Work out the finished part from the listing and answer in its coordinate system (mm). Coordinates: 2 decimals unless noted, no trailing zeros. Order: outer loops, then holes, each group sorted by start corner. A loop starts at its lowest first (then second) coordinate and runs counter-clockwise, first axis right, second up. Notation, with made-up numbers: M -34.75,-35.5 L 3.25,-35.5 A12 ccw 3.25,-16.5 Z; hole C 61,88 d7. An arc over 180 degrees is marked long. Use a Markdown table: item, result. Add a question column.
from build123d import *

# Parameters (mm, degrees)
SKETCH1_W           = 600
SKETCH1_H           = 300
BOSS_EXTRUDE1_DEPTH = 3
SKETCH2_R           = 82.5
SKETCH2_R_2         = 6.5
SKETCH2_W           = 30
SKETCH2_H           = 3
SKETCH2_W_2         = 3
SKETCH2_H_2         = 30
CUT_EXTRUDE2_DEPTH  = 5
SKETCH3_W           = 175.2
SKETCH3_H           = 3.2
CUT_EXTRUDE3_DEPTH  = 10


with BuildPart() as part:
    # Sketch1 → Boss-Extrude1 (new body)
    with BuildSketch(Plane(origin=(0, 0, 0), x_dir=(1, 0, 0), z_dir=(0, 1, 0))):
        with Locations((300, 150)):
            Rectangle(SKETCH1_W, SKETCH1_H)
    extrude(amount=BOSS_EXTRUDE1_DEPTH)

    # Sketch2 → Cut-Extrude2 (cut)
    with BuildSketch(Plane(origin=(0, 3, 0), x_dir=(1, 0, 0), z_dir=(0, 1, 0))):
        with Locations(Location((115, 150, 0), (0, 0, 270))):
            Circle(SKETCH2_R)
        with Locations(Location((263.5, 150, 0), (0, 0, 270))):
            Circle(SKETCH2_R_2)
        with Locations(Location((336.5, 150, 0), (0, 0, 90))):
            Circle(SKETCH2_R_2)
        with Locations(Location((485, 150, 0), (0, 0, 90))):
            Circle(SKETCH2_R)
        with Locations((90, 1.5)):
            Rectangle(SKETCH2_W, SKETCH2_H)
        with Locations((30, 1.5)):
            Rectangle(SKETCH2_W, SKETCH2_H)
        with Locations((150, 1.5)):
            Rectangle(SKETCH2_W, SKETCH2_H)
        with Locations((210, 1.5)):
            Rectangle(SKETCH2_W, SKETCH2_H)
        with Locations((270, 1.5)):
            Rectangle(SKETCH2_W, SKETCH2_H)
        with Locations((330, 1.5)):
            Rectangle(SKETCH2_W, SKETCH2_H)
        with Locations((390, 1.5)):
            Rectangle(SKETCH2_W, SKETCH2_H)
        with Locations((450, 1.5)):
            Rectangle(SKETCH2_W, SKETCH2_H)
        with Locations((510, 1.5)):
            Rectangle(SKETCH2_W, SKETCH2_H)
        with Locations((570, 1.5)):
            Rectangle(SKETCH2_W, SKETCH2_H)
        with Locations((570, 298.5)):
            Rectangle(SKETCH2_W, SKETCH2_H)
        with Locations((510, 298.5)):
            Rectangle(SKETCH2_W, SKETCH2_H)
        with Locations((450, 298.5)):
            Rectangle(SKETCH2_W, SKETCH2_H)
        with Locations((390, 298.5)):
            Rectangle(SKETCH2_W, SKETCH2_H)
        with Locations((330, 298.5)):
            Rectangle(SKETCH2_W, SKETCH2_H)
        with Locations((270, 298.5)):
            Rectangle(SKETCH2_W, SKETCH2_H)
        with Locations((210, 298.5)):
            Rectangle(SKETCH2_W, SKETCH2_H)
        with Locations((150, 298.5)):
            Rectangle(SKETCH2_W, SKETCH2_H)
        with Locations((90, 298.5)):
            Rectangle(SKETCH2_W, SKETCH2_H)
        with Locations((30, 298.5)):
            Rectangle(SKETCH2_W, SKETCH2_H)
        with Locations((1.5, 210)):
            Rectangle(SKETCH2_W_2, SKETCH2_H_2)
        with Locations((1.5, 270)):
            Rectangle(SKETCH2_W_2, SKETCH2_H_2)
        with Locations((1.5, 150)):
            Rectangle(SKETCH2_W_2, SKETCH2_H_2)
        with Locations((1.5, 90)):
            Rectangle(SKETCH2_W_2, SKETCH2_H_2)
        with Locations((1.5, 30)):
            Rectangle(SKETCH2_W_2, SKETCH2_H_2)
        with Locations((598.5, 30)):
            Rectangle(SKETCH2_W_2, SKETCH2_H_2)
        with Locations((598.5, 90)):
            Rectangle(SKETCH2_W_2, SKETCH2_H_2)
        with Locations((598.5, 150)):
            Rectangle(SKETCH2_W_2, SKETCH2_H_2)
        with Locations((598.5, 210)):
            Rectangle(SKETCH2_W_2, SKETCH2_H_2)
        with Locations((598.5, 270)):
            Rectangle(SKETCH2_W_2, SKETCH2_H_2)
    extrude(amount=-CUT_EXTRUDE2_DEPTH, mode=Mode.SUBTRACT)

    # Sketch3 → Cut-Extrude3 (cut)
    with BuildSketch(Plane(origin=(0, 3, 0), x_dir=(1, 0, 0), z_dir=(0, 1, 0))):
        with Locations((300, 280.2)):
            Rectangle(SKETCH3_W, SKETCH3_H)
    extrude(amount=-CUT_EXTRUDE3_DEPTH, mode=Mode.SUBTRACT)


solid = part.part
(1) A cutting plane is placed at A-A on x = 485. Write down the section's boundary in (y, z).
(2) The mould has two halves that part along Z. Classify faces 1 (the cylindrical face through (259.545, 1.521, -155.158)), 2 (the flat face through (296, 0, -152)): pulls with the +Z half, pulls with the -Z half, needs draft (parallel to the pull), parting line crosses it, or undercut.
(3) Given P1, Ø1.5, axis at y = 1, z = -276, coming from the +X side; P2, Ø1.5, axis at x = 538.5, y = 2.5, coming from the +Z side; P3, Ø1.5, axis at x = 94.5, y = 1, coming from the +Z side; P4, Ø0.9, axis at x = 570, y = 2, coming from the -Z side, each flat-ended and moving along its own axis, determine where each tip first touches the part or whether it passes through.
(4) A cutting plane is placed at B-B on z = -150. Write down the section's boundary in (x, y).
(5) A cutting plane is placed at C-C on x = 263.5. Write down the section's boundary in (y, z), plus the area to 3 significant figures.
(6) Straight lines are drawn through the part: line 1 (X direction, y = 1.1, z = -150); line 2 (Z direction, x = 263.5, y = 2.35); line 3 (X direction, y = 2.95, z = -122). For each, find the intervals that lie inside material, in ascending order.
(7) A cutting plane is placed at D-D on z = -188.5. Write down the section's boundary in (x, y), plus the area to 3 significant figures.
From the geometry:
| question | item | result |
|---|---|---|
| 1 | outline | M 0,-300 L 3,-300 L 3,-232.5 L 0,-232.5 Z; M 0,-67.5 L 3,-67.5 L 3,0 L 0,0 Z |
| 2 | face 1 | undercut |
| 2 | face 2 | needs draft |
| 3 | P1 | stops at x = 597 |
| 3 | P2 | stops at z = 0 |
| 3 | P3 | stops at z = -3 |
| 3 | P4 | stops at z = -297 |
| 4 | outline | M 3,0 L 32.5,0 L 32.5,3 L 3,3 Z; M 197.5,0 L 257,0 L 257,3 L 197.5,3 Z; M 270,0 L 330,0 L 330,3 L 270,3 Z; M 343,0 L 402.5,0 L 402.5,3 L 343,3 Z; M 567.5,0 L 597,0 L 597,3 L 567.5,3 Z |
| 5 | outline | M 0,-297 L 3,-297 L 3,-281.8 L 0,-281.8 Z; M 0,-278.6 L 3,-278.6 L 3,-156.5 L 0,-156.5 Z; M 0,-143.5 L 3,-143.5 L 3,-3 L 0,-3 Z |
| 5 | area | 833 mm2 |
| 6 | line 1 | x = 3 to 32.5, 197.5 to 257, 270 to 330, 343 to 402.5, 567.5 to 597 |
| 6 | line 2 | z = -297 to -281.8, -278.6 to -156.5, -143.5 to -3 |
| 6 | line 3 | x = 0 to 37.4, 192.6 to 407.4, 562.6 to 600 |
| 7 | outline | M 0,0 L 42.03,0 L 42.03,3 L 0,3 Z; M 187.97,0 L 412.03,0 L 412.03,3 L 187.97,3 Z; M 557.97,0 L 600,0 L 600,3 L 557.97,3 Z |
| 7 | area | 924 mm2 |
